Autodesk Inventor part; units mm, degrees
ref_plane "Work Plane1" through (0, 0, -1.15) normal (0, 0, -1) x (-1, 0, 0)
ref_plane "YZ Plane" through (0, 0, 0) normal (1, 0, 0) x (0, 1, 0)
ref_plane "XZ Plane" through (0, 0, 0) normal (0, 1, 0) x (-1, 0, 0)
sketch "Sketch1" plane through (0, 0, 0) normal (0, 0, 1) x (1, 0, 0)
  line L0 (0, 0) -> (1.6, 0) construction
  circle A0 centre (0, 0) radius 2.5
  circle A1 centre (0, 0) radius 3
  arc A2 (0, 3.7) -> (-3.7, 0) centre (0, 0) ccw
  line L1 (0, 0) -> (0, 3.7) construction
  line L2 (0, 3.7) -> (0, 3.7)
  arc A3 (3.7, 0) -> (0, 3.7) centre (0, 0) ccw
  line L3 (0, 0) -> (0, 0) construction
  line L4 (0, 0) -> (-3.7, 0) construction
  line L5 (-3.7, 0) -> (-3.7, -16)
  arc A4 (-3.7, -16) -> (0, -19.7) centre (0, -16) ccw
  line L6 (0, -19.7) -> (0, -19.7)
  arc A5 (0, -19.7) -> (3.7, -16) centre (0, -16) ccw
  line L7 (3.7, -16) -> (3.7, 0)
  dimension "x" = 1.6
  dimension "d1" = 5
  dimension "d2" = 6
  dimension "d3" = 3.7
  dimension "d4" = 0
  dimension "d17" = 16
extrude "Extrusion1" add sketch "Sketch1" along normal mid plane 3.9 contours A0 | A1 | A3 L7 A5 A4 L5 A2
extrude "Extrusion2" cut sketch "Sketch1" against normal up to surface (3.9 mm away) from surface at 1.95 contours A0 | A1
extrude "Extrusion3" add sketch "Sketch1" along normal mid plane 2.4 contours A1
pattern_linear "Rectangular Pattern1" count 3 spacing -8 along (0, 1, 0) of "Extrusion2", "Extrusion3"
ref_plane "Work Plane1" through (0, 0, -1.15) normal (0, 0, -1) x (-1, 0, 0)
extrude "Extrusion4" add sketch "Sketch1" along normal up to surface (0.05 mm away) from surface at -1.2 contours A0 | A1 | A3 L7 A5 A4 L5 A2
equation "\"d13\" = 5 * x"
equation "\"d20\" = -5 * x"
properties part number "LEGO technic thin liftarm"
Design review of the part built by this model. Coordinates are the model's own, in mm. A direction names the side the tool comes from. Round coordinates to 2 decimals unless told otherwise and drop trailing zeros. Order: outer loops, then holes, each group sorted by start corner. A loop starts at its lowest first (then second) coordinate and runs counter-clockwise, first axis right, second up. Notation, with made-up numbers: M 26,-29 L 83,-29 A4 ccw 83,-22 Z; hole C -12,-34.75 d3. An arc over 180 degrees is marked long. Answer as CSV lines item,"result". Start each with the question number.
1) The part is to be moulded in two halves that separate along Y. For faces 4 (the face through (-0.1, 3.7, 0)), 5 (the face through (-0.54, -5.56, 0.01)), 6 (the face through (3.7, -8, 0)), say which applies: +Y half, -Y half, draft (parallel to the pull), parting line (faces both ways), or undercut.
2) For pin 1 Ø1.8 at (x, y) = (0, -8.5) entering from -Z; pin 2 Ø1.5 at (x, y) = (-0.5, -16.5) entering from +Z; pin 3 Ø3 at (x, y) = (-1, -6.5) entering from +Z; pin 4 Ø2 at (x, z) = (-2.5, -0.5) entering from +Y, all flat-tipped, find the tip position at first contact; note any pin that passes through.
3) Add section A-A (y = -8). Give the boundary of the cut face in (x, z), then the cut area to 3 significant figures.
4) Tool access review of faces 1 (the face through (-2, -5, 1.95)), 2 (the face through (-2, -6, 1.2)), 3 (the face through (-0.391, -5.026, -1.57)): name each direction out of +Z, -Z, +X, -X, +Y, -Y from which nothing blocks a thin tool from reaching the whole face with its end or side.
5) Add section B-B (y = 1.5). Give the boundary of the cut face in (x, z), then the cut area to 3 significant figures.
6) Wall thickness on line 1 along Y through (x, z) = (0, -1.75); line 2 along X through (y, z) = (0, -0.3); line 3 along Y through (x, z) = (-0.75, 0.85): over which ranges is each line inside the solid? List them lowest first. Write a range as [from, to].
Resolved:
1,face 4,"+Y half"
1,face 5,"undercut"
1,face 6,"draft"
2,pin 1,"z = -1.2"
2,pin 2,"z = -1.15"
2,pin 3,"z = 1.95"
2,pin 4,"y = 3.38"
3,outline,"M -3.7,-1.95 L -3,-1.95 L -3,-1.2 L 3,-1.2 L 3,-1.95 L 3.7,-1.95 L 3.7,1.95 L 3,1.95 L 3,1.2 L 2.5,1.2 L 2.5,-1.15 L -2.5,-1.15 L -2.5,1.2 L -3,1.2 L -3,1.95 L -3.7,1.95 Z"
3,area,"8.11 mm^2"
4,face 1,"+Z, +X, -X, +Y, -Y"
4,face 2,"+Z"
4,face 3,"-Z"
5,outline,"M -3.38,-1.95 L -2.6,-1.95 L -2.6,-1.2 L 2.6,-1.2 L 2.6,-1.95 L 3.38,-1.95 L 3.38,1.95 L 2.6,1.95 L 2.6,1.2 L 2,1.2 L 2,-1.15 L -2,-1.15 L -2,1.2 L -2.6,1.2 L -2.6,1.95 L -3.38,1.95 Z"
5,area,"9.19 mm^2"
6,line 1,"[-19.7, -19], [-13, -11], [-5, -3], [3, 3.7]"
6,line 2,"[-3.7, -2.5], [2.5, 3.7]"
6,line 3,"[-19.62, -18.38], [-13.62, -10.38], [-5.62, -2.38], [2.38, 3.62]"
